Verification items for the finished model (mm, model axes). Face numbers are marked on the shaded views. A direction names the side the tool comes from. Coordinates: 2 decimals unless noted, no trailing zeros. Order: outer loops, then holes, each group sorted by start corner. A loop starts at its lowest first (then second) coordinate and runs counter-clockwise, first axis right, second up. Notation, with made-up numbers: (33.25, -15.75) -> (86.25, -15.75) arc R32 ccw to (86.25, 14.25) -> close; hole circle Ø9 at (-26, 46). An arc over 180 degrees is marked (long way). Write item = value, one per line. Start each with the question number.
from build123d import *

# Parameters (mm, degrees)
SKETCH1_R           = 1.3
BOSS_EXTRUDE1_DEPTH = 4


with BuildPart() as part:
    # Sketch1 → Boss-Extrude1 (new body)
    with BuildSketch(Plane.XY):
        with BuildLine():
            Line((10.823243212, 2.571433572), (5, 4.435742065))
            ThreePointArc((5, 4.435742065), (2.74093184, 4.97035983), (0.426426599, 5.15))
            Line((0.426426599, 5.15), (-0.426426599, 5.15))
            ThreePointArc((-0.426426599, 5.15), (-2.74093184, 4.97035983), (-5, 4.435742065))
            Line((-5, 4.435742065), (-10.823243212, 2.571433572))
            ThreePointArc((-10.823243212, 2.571433572), (-12.7, 0), (-10.823243212, -2.571433572))
            Line((-10.823243212, -2.571433572), (-5, -4.435742065))
            ThreePointArc((-5, -4.435742065), (-2.74093184, -4.97035983), (-0.426426599, -5.15))
            Line((-0.426426599, -5.15), (0.426426599, -5.15))
            ThreePointArc((0.426426599, -5.15), (2.74093184, -4.97035983), (5, -4.435742065))
            Line((5, -4.435742065), (10.823243212, -2.571433572))
            ThreePointArc((10.823243212, -2.571433572), (12.7, 0), (10.823243212, 2.571433572))
        make_face()
        with Locations((10, 0)):
            Circle(SKETCH1_R, mode=Mode.SUBTRACT)
        with Locations(Location((-10, 0, 0), (0, 0, 180))):
            Circle(SKETCH1_R, mode=Mode.SUBTRACT)
        Polygon((2.165063509, 3.75), (-2.165063509, 3.75), (-4.330127019, 0), (-2.165063509, -3.75), (2.165063509, -3.75), (4.330127019, 0), align=None, mode=Mode.SUBTRACT)
    extrude(amount=BOSS_EXTRUDE1_DEPTH)


solid = part.part
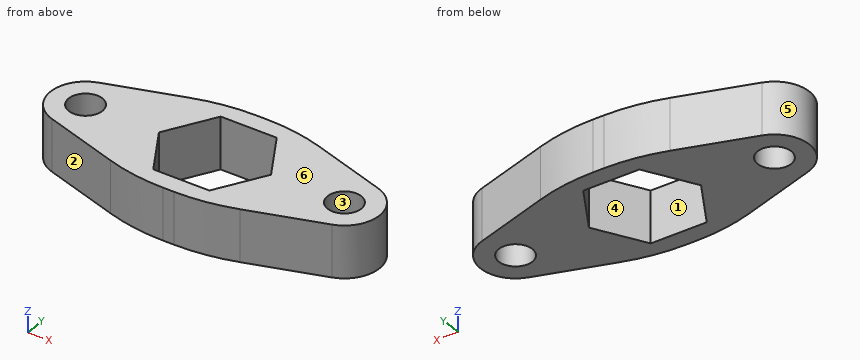
Item 1: Section check A-A (z = 2.6). Record the boundary of the cut face in (x, y), then the cut area to 3 significant figures.
Item 2: Gauge pin test, flat end, axial feed: P1, Ø4, axis at x = 4, y = 0, coming from the -Z side. Record the tip position at first contact, or that the pin passes through.
Item 3: Section check B-B (x = -1.5). Record the boundary of the cut face in (y, z).
Item 4: Tool access check on the marked faces 1 and 2. Record the directions out of +Z, -Z, +X, -X, +Y, -Y that give a thin tool (end or side, any length) a straight path to the whole face; none if there is none.
Item 5: Section check D-D (x = 7.75). Record the boundary of the cut face in (y, z).
Item 6: Thickness scan on line 1 (X direction, y = -0.75, z = 3); line 2 (X direction, y = -0.5, z = 1.75); line 3 (Y direction, x = -10, z = 1.8) (3 decimals). Record the ranges inside material, lowest first.
Item 7: Mould release check, pull along X, two halves, no side actions. Record for the marked faces 3, 4, 5 and 6: pulls with the +X half, pulls with the -X half, needs draft (parallel to the pull), parting line crosses it, or undercut.
Item 8: Section check C-C (y = 3.5). Record the boundary of the cut face in (x, z), then the cut area to 3 significant figures.
Filled sheet:
q1.outline = (-10.82, -2.57) -> (-5, -4.44) arc R15 ccw to (-0.43, -5.15) -> (0.43, -5.15) arc R15 ccw to (5, -4.44) -> (10.82, -2.57) arc R2.7 ccw to (10.82, 2.57) -> (5, 4.44) arc R15 ccw to (0.43, 5.15) -> (-0.43, 5.15) arc R15 ccw to (-5, 4.44) -> (-10.82, 2.57) arc R2.7 ccw to start; hole circle Ø2.6 at (-10, 0); hole (-4.33, 0) -> (-2.17, -3.75) -> (2.17, -3.75) -> (4.33, 0) -> (2.17, 3.75) -> (-2.17, 3.75) -> close; hole circle Ø2.6 at (10, 0)
q1.area = 135 mm^2
q2.P1 = 0
q3.outline = (-5.11, 0) -> (-3.75, 0) -> (-3.75, 4) -> (-5.11, 4) -> close; (3.75, 0) -> (5.11, 0) -> (5.11, 4) -> (3.75, 4) -> close
q4.face_1 = +Z, -Z
q4.face_2 = +Z, -Z, -X, -Y
q5.outline = (-3.56, 0) -> (3.56, 0) -> (3.56, 4) -> (-3.56, 4) -> close
q6.line_1 = -12.59 to -11.06, -8.94 to -3.9, 3.9 to 8.94, 11.06 to 12.59
q6.line_2 = -12.65 to -11.2, -8.8 to -4.04, 4.04 to 8.8, 11.2 to 12.65
q6.line_3 = -2.835 to -1.3, 1.3 to 2.835
q7.face_3 = undercut
q7.face_4 = undercut
q7.face_5 = pulls with the -X half
q7.face_6 = needs draft
q8.outline = (-7.92, 0) -> (-2.31, 0) -> (-2.31, 4) -> (-7.92, 4) -> close; (2.31, 0) -> (7.92, 0) -> (7.92, 4) -> (2.31, 4) -> close
q8.area = 44.9 mm^2
